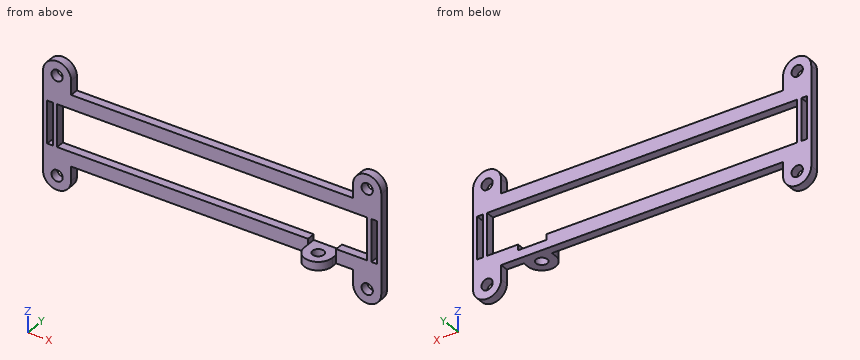
```python
from build123d import *

# Parameters (mm, degrees)
SKETCH1_R           = 5
SKETCH1_R_2         = 2
SKETCH1_W           = 120
SKETCH1_H           = 25
SKETCH1_W_2         = 110
SKETCH1_H_2         = 15
BOSS_EXTRUDE1_DEPTH = 3
SKETCH2_W           = 2
SKETCH2_H           = 15
CUT_EXTRUDE1_DEPTH  = 3
SKETCH3_R           = 2
BOSS_EXTRUDE3_DEPTH = 3
SKETCH4_W           = 10
SKETCH4_H           = 3
CUT_EXTRUDE2_DEPTH  = 2


with BuildPart() as part:
    # Sketch1 → Boss-Extrude1 (new body)
    # profile 1 of 13: a face of its own
    with BuildSketch(Plane(origin=(0, 0, 0), x_dir=(1, 0, 0), z_dir=(0, 1, 0))):
        with Locations((5, 30)):
            Circle(SKETCH1_R)
        with Locations(Location((5, 30, 0), (0, 0, 270))):
            Circle(SKETCH1_R_2, mode=Mode.SUBTRACT)
    # profile 2 of 13: a face of its own
    with BuildSketch(Plane(origin=(0, 0, 0), x_dir=(1, 0, 0), z_dir=(0, 1, 0))):
        with BuildLine():
            Line((0, 30), (0, 25))
            Line((0, 25), (5, 25))
            ThreePointArc((5, 25), (1.464466094, 26.464466094), (0, 30))
        make_face()
    # profile 3 of 13: a face of its own
    with BuildSketch(Plane(origin=(0, 0, 0), x_dir=(1, 0, 0), z_dir=(0, 1, 0))):
        with BuildLine():
            ThreePointArc((10, 30), (8.535533906, 26.464466094), (5, 25))
            Line((5, 25), (10, 25))
            Line((10, 25), (10, 30))
        make_face()
    # profile 4 of 13: a face of its own
    with BuildSketch(Plane(origin=(0, 0, 0), x_dir=(1, 0, 0), z_dir=(0, 1, 0))):
        with Locations((60, 12.5)):
            Rectangle(SKETCH1_W, SKETCH1_H)
        with Locations((60, 12.5)):
            Rectangle(SKETCH1_W_2, SKETCH1_H_2, mode=Mode.SUBTRACT)
    # profile 5 of 13: a face of its own
    with BuildSketch(Plane(origin=(0, 0, 0), x_dir=(1, 0, 0), z_dir=(0, 1, 0))):
        with BuildLine():
            Line((5, 0), (0, 0))
            Line((0, 0), (0, -5))
            ThreePointArc((0, -5), (1.464466094, -1.464466094), (5, 0))
        make_face()
    # profile 6 of 13: a face of its own
    with BuildSketch(Plane(origin=(0, 0, 0), x_dir=(1, 0, 0), z_dir=(0, 1, 0))):
        with BuildLine():
            Line((10, 0), (5, 0))
            ThreePointArc((5, 0), (8.535533906, -1.464466094), (10, -5))
            Line((10, -5), (10, 0))
        make_face()
    # profile 7 of 13: a face of its own
    with BuildSketch(Plane(origin=(0, 0, 0), x_dir=(1, 0, 0), z_dir=(0, 1, 0))):
        with Locations((5, -5)):
            Circle(SKETCH1_R)
        with Locations(Location((5, -5, 0), (0, 0, 270))):
            Circle(SKETCH1_R_2, mode=Mode.SUBTRACT)
    # profile 8 of 13: a face of its own
    with BuildSketch(Plane(origin=(0, 0, 0), x_dir=(1, 0, 0), z_dir=(0, 1, 0))):
        with BuildLine():
            Line((110, 30), (110, 25))
            Line((110, 25), (115, 25))
            ThreePointArc((115, 25), (111.464466094, 26.464466094), (110, 30))
        make_face()
    # profile 9 of 13: a face of its own
    with BuildSketch(Plane(origin=(0, 0, 0), x_dir=(1, 0, 0), z_dir=(0, 1, 0))):
        with Locations((115, 30)):
            Circle(SKETCH1_R)
        with Locations(Location((115, 30, 0), (0, 0, 270))):
            Circle(SKETCH1_R_2, mode=Mode.SUBTRACT)
    # profile 10 of 13: a face of its own
    with BuildSketch(Plane(origin=(0, 0, 0), x_dir=(1, 0, 0), z_dir=(0, 1, 0))):
        with BuildLine():
            ThreePointArc((120, 30), (118.535533906, 26.464466094), (115, 25))
            Line((115, 25), (120, 25))
            Line((120, 25), (120, 30))
        make_face()
    # profile 11 of 13: a face of its own
    with BuildSketch(Plane(origin=(0, 0, 0), x_dir=(1, 0, 0), z_dir=(0, 1, 0))):
        with BuildLine():
            Line((115, 0), (110, 0))
            Line((110, 0), (110, -5))
            ThreePointArc((110, -5), (111.464466094, -1.464466094), (115, 0))
        make_face()
    # profile 12 of 13: a face of its own
    with BuildSketch(Plane(origin=(0, 0, 0), x_dir=(1, 0, 0), z_dir=(0, 1, 0))):
        with BuildLine():
            Line((120, 0), (115, 0))
            ThreePointArc((115, 0), (118.535533906, -1.464466094), (120, -5))
            Line((120, -5), (120, 0))
        make_face()
    # profile 13 of 13: a face of its own
    with BuildSketch(Plane(origin=(0, 0, 0), x_dir=(1, 0, 0), z_dir=(0, 1, 0))):
        with Locations((115, -5)):
            Circle(SKETCH1_R)
        with Locations(Location((115, -5, 0), (0, 0, 270))):
            Circle(SKETCH1_R_2, mode=Mode.SUBTRACT)
    extrude(amount=BOSS_EXTRUDE1_DEPTH)

    # Sketch2 → Cut-Extrude1 (cut)
    with BuildSketch(Plane(origin=(0, 3, 0), x_dir=(1, 0, 0), z_dir=(0, 1, 0))):
        with Locations((117.5, 12.5)):
            Rectangle(SKETCH2_W, SKETCH2_H)
        with Locations((2.5, 12.5)):
            Rectangle(SKETCH2_W, SKETCH2_H)
    extrude(amount=-CUT_EXTRUDE1_DEPTH, mode=Mode.SUBTRACT)

    # Sketch3 → Boss-Extrude3 (add)
    # profile 1 of 3: a face of its own
    with BuildSketch(Plane(origin=(0, 0, -25), x_dir=(-1, 0, 0), z_dir=(0, 0, -1))):
        with BuildLine():
            ThreePointArc((-103.578198336, 0), (-103.893413516, -0.98310947), (-104, -2.01))
            ThreePointArc((-104, -2.01), (-99, -7.01), (-94, -2.01))
            ThreePointArc((-94, -2.01), (-94.106586484, -0.98310947), (-94.421801664, 0))
            Line((-94.421801664, 0), (-103.578198336, 0))
        make_face()
        with Locations((-99, -2.01)):
            Circle(SKETCH3_R, mode=Mode.SUBTRACT)
    # profile 2 of 3: a face of its own
    with BuildSketch(Plane(origin=(0, 0, -25), x_dir=(-1, 0, 0), z_dir=(0, 0, -1))):
        with BuildLine():
            ThreePointArc((-94.421801664, 0), (-94.106586484, -0.98310947), (-94, -2.01))
            Line((-94, -2.01), (-94, 0))
            Line((-94, 0), (-94.421801664, 0))
        make_face()
    # profile 3 of 3: a face of its own
    with BuildSketch(Plane(origin=(0, 0, -25), x_dir=(-1, 0, 0), z_dir=(0, 0, -1))):
        with BuildLine():
            Line((-104, 0), (-104, -2.01))
            ThreePointArc((-104, -2.01), (-103.893413516, -0.98310947), (-103.578198336, 0))
            Line((-103.578198336, 0), (-104, 0))
        make_face()
    extrude(amount=-BOSS_EXTRUDE3_DEPTH)

    # Sketch4 → Cut-Extrude2 (cut)
    with BuildSketch(Plane.XY.offset(-20)):
        with Locations((99, 1.5)):
            Rectangle(SKETCH4_W, SKETCH4_H)
    extrude(amount=-CUT_EXTRUDE2_DEPTH, mode=Mode.SUBTRACT)


solid = part.part
```
Input: part model. Units: mm. Frame: model coordinates. Coordinates: 2 decimals unless noted, no trailing zeros. Write each loop counter-clockwise with the first axis right and the second up, starting at its lowest first coordinate (ties: lowest second). Pieces come first, ordered by that corner, then holes. Notation, with made-up numbers: (-19, 1) -> (38, 1) arc R18 cw to (38, 19) -> close; hole circle Ø6 at (-21, 56). An arc over 180 degrees is marked (long way). Answer as a JSON object with one key per item and string values.
1. Section B-B on z = -15.5. Return the cut outline in (x, y), then the cut area to 3 significant figures.
Result set:
{"outline": "(0, 0) -> (1.5, 0) -> (1.5, 3) -> (0, 3) -> close; (3.5, 0) -> (5, 0) -> (5, 3) -> (3.5, 3) -> close; (115, 0) -> (116.5, 0) -> (116.5, 3) -> (115, 3) -> close; (118.5, 0) -> (120, 0) -> (120, 3) -> (118.5, 3) -> close", "area": "18.0 mm2"}
2. First-contact query: P1, Ø1.6, axis at x = 3, y = 1.5, coming from the +Z side; P2, Ø10, axis at x = 85.5, z = 0.5, coming from the +Y side; P3, Ø3, axis at x = 93, z = -23.5, coming from the -Y side; P4, Ø22.5, axis at x = 41, z = -6, coming from the -Y side. Flat tips, straight axial feed; report the tip coordinate or a pass-through.
Result set:
{"P1": "stops at z = 9.85", "P2": "stops at y = 3", "P3": "stops at y = -4.19", "P4": "stops at y = 0"}
3. Section A-A on x = 99. Return the cut outline in (y, z).
Result set:
{"outline": "(-7.01, -25) -> (-4.01, -25) -> (-4.01, -22) -> (-7.01, -22) -> close; (-0.01, -25) -> (3, -25) -> (3, -22) -> (-0.01, -22) -> close; (0, -5) -> (3, -5) -> (3, 0) -> (0, 0) -> close"}
4. Section C-C on x = 82. Return the cut outline in (y, z).
Result set:
{"outline": "(0, -25) -> (3, -25) -> (3, -20) -> (0, -20) -> close; (0, -5) -> (3, -5) -> (3, 0) -> (0, 0) -> close"}
5. Material intervals for line 1 (X direction, y = 1.9, z = 5); line 2 (Y direction, x = 99, z = -23); line 3 (Y direction, x = 38, z = -1), sorted ascending. Write a range as from..to.
Result set:
{"line 1": "x = 0..3, 7..10, 110..113, 117..120", "line 2": "y = -7.01..-4.01, -0.01..3", "line 3": "y = 0..3"}
